from build123d import *

# Parameters (mm, degrees)
BOSS_EXTRUDE1_DEPTH = 300
SKETCH6_W           = 25
SKETCH6_H           = 25
BOSS_EXTRUDE2_DEPTH = 100


with BuildPart() as part:
    # Sketch3 → Boss-Extrude1 (new body)
    with BuildSketch(Plane(origin=(0, 0, 0), x_dir=(0, 0, -1), z_dir=(1, 0, 0))):
        Polygon((-476.395417156, 336.925610034), (-411.69065588, 578.407066606), (-431.009172406, 583.583447508), (-491.741956916, 356.925610034), (-776.395417156, 356.925610034), (-776.395417156, 336.925610034), align=None)
    extrude(amount=BOSS_EXTRUDE1_DEPTH)

    # Sketch6 → Boss-Extrude2 (add)
    with BuildSketch(Plane.XZ.offset(-336.925610034)):
        with Locations((277.5, 753.895417156)):
            Rectangle(SKETCH6_W, SKETCH6_H)
        with Locations((22.5, 753.895417156)):
            Rectangle(SKETCH6_W, SKETCH6_H)
        with Locations((277.5, 498.895417156)):
            Rectangle(SKETCH6_W, SKETCH6_H)
        with Locations((22.5, 498.895417156)):
            Rectangle(SKETCH6_W, SKETCH6_H)
    extrude(amount=BOSS_EXTRUDE2_DEPTH)


solid = part.part
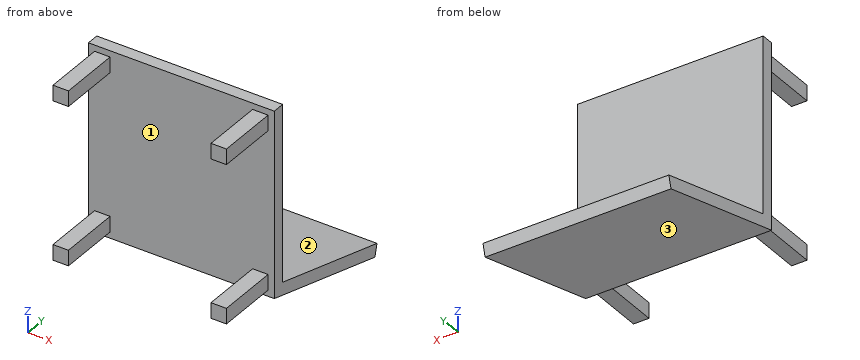
Geometry: final body of the model. Coordinates: model frame, mm. Face numbers are marked on the shaded views. Give positions to 0.01 mm unless a question says otherwise; leave off trailing zeros. Write each loop counter-clockwise with the first axis right and the second up, starting at its lowest first coordinate (ties: lowest second). Pieces come first, ordered by that corner, then holes. Notation, with made-up numbers: M 22.5,89.25 L 72.5,89.25 A18 cw 72.5,95.25 Z; hole C 57.25,85 d6. An arc over 180 degrees is marked long. Answer in a Markdown table with one row per item. Add a question column.
(1) Mould query, pull axis Z, two halves, no side actions, for the marked faces 1, 2 and 3. Classes: +Z half, -Z half, draft (parallel to the pull), parting line (faces both ways), or undercut.
(2) Section C-C on x = 24.5. Return loops of the section in (y, z), and give its area (3 significant figures).
(3) Section A-A on x = 211.5. Return loops of the section in (y, z).
(4) Section D-D on y = 453. Return loops of the section in (x, z), and give its area (3 significant figures).
(5) First-contact query: pin 1 (20 mm diameter, centred on y = 304.5, z = 495, fed in from -X); pin 2 (20 mm diameter, centred on x = 271.5, y = 310, fed in from -Z); pin 3 (20 mm diameter, centred on y = 263.5, z = 502, fed in from +X); pin 4 (1 mm diameter, centred on y = 358.5, z = 645, fed in from -X). Flat tips, straight axial feed; report the tip coordinate or a pass-through.
(6) Ray query, line 1 (X direction, y = 280, z = 752); line 2 (Z direction, x = 285, y = 329.5); line 3 (Y direction, x = 14.5, z = 537). Return the intervals inside material, ascending.
(7) Section B-B on z = 592.5. Return loops of the section in (x, y), and give its area (3 significant figures).
Result set:
| question | item | result |
|---|---|---|
| 1 | face 1 | undercut |
| 1 | face 2 | +Z half |
| 1 | face 3 | -Z half |
| 2 | outline | M 236.93,486.4 L 336.93,486.4 L 336.93,476.4 L 578.41,411.69 L 583.58,431.01 L 356.93,491.74 L 356.93,776.4 L 336.93,776.4 L 336.93,766.4 L 236.93,766.4 L 236.93,741.4 L 336.93,741.4 L 336.93,511.4 L 236.93,511.4 Z |
| 2 | area | 15,700 mm^2 |
| 3 | outline | M 336.93,476.4 L 578.41,411.69 L 583.58,431.01 L 356.93,491.74 L 356.93,776.4 L 336.93,776.4 Z |
| 4 | outline | M 0,445.29 L 300,445.29 L 300,466 L 0,466 Z |
| 4 | area | 6,210 mm^2 |
| 5 | pin 1 | stops at x = 10 |
| 5 | pin 2 | stops at z = 486.4 |
| 5 | pin 3 | stops at x = 290 |
| 5 | pin 4 | passes through |
| 6 | line 1 | x = 10 to 35, 265 to 290 |
| 6 | line 2 | z = 486.4 to 511.4, 741.4 to 766.4 |
| 6 | line 3 | y = 336.93 to 356.93 |
| 7 | outline | M 0,336.93 L 300,336.93 L 300,356.93 L 0,356.93 Z |
| 7 | area | 6,000 mm^2 |
